Autodesk Inventor part; units mm, degrees
ref_plane "YZ Plane" through (0, 0, 0) normal (1, 0, 0) x (0, 1, 0)
ref_plane "XZ Plane" through (0, 0, 0) normal (0, 1, 0) x (-1, 0, 0)
ref_plane "XY Plane" through (0, 0, 0) normal (0, 0, 1) x (1, 0, 0)
sketch "Sketch1" plane through (0, 0, 0) normal (0, 1, 0) x (-1, 0, 0)
  line L0 (0, 0) -> (-25.4, 0)
  line L1 (-25.4, 0) -> (-25.4, 25.4)
  line L2 (-25.4, 25.4) -> (0, 25.4)
  line L3 (0, 25.4) -> (0, 0)
  line L4 (-1.5875, 23.8125) -> (-23.8125, 23.8125)
  line L5 (-23.8125, 23.8125) -> (-23.8125, 1.5875)
  line L6 (-23.8125, 1.5875) -> (-1.5875, 1.5875)
  line L7 (-1.5875, 1.5875) -> (-1.5875, 23.8125)
  dimension "d0" = 25.4
  dimension "d2" = 25.4
  dimension "d3" = 1.5875
extrude "Extrusion1" add sketch "Sketch1" along normal blind 593.725
sketch "Sketch5" plane through (25.4, 0, 25.4) normal (1, 0, 0) x (0, 0, -1)
  circle A0 centre (12.7, 561.975) radius 3.3782
  circle A1 centre (12.7, 539.75) radius 3.3782
  circle A2 centre (12.7, 454.025) radius 3.3782
extrude "Cut3" cut sketch "Sketch5" against normal blind 2540
sketch "Sketch6" plane through (0, 0, 25.4) normal (0, 0, 1) x (1, 0, 0)
  circle A0 centre (12.7, 428.625) radius 3.3782
  circle A1 centre (12.7, 377.825) radius 3.3782
  circle A2 centre (12.7, 571.5) radius 3.3782
  circle A3 centre (12.7, 549.275) radius 3.3782
extrude "Cut4" cut sketch "Sketch6" against normal blind 2540
equation "\"BendRadius\" = Thickness"
equation "\"BendReliefWidth\" = Thickness"
equation "\"BendReliefDepth\" = 0.5 * Thickness"
equation "\"CornerReliefSize\" = 4 * Thickness"
equation "\"MinimumRemnant\" = 2 * Thickness"
equation "\"TransitionRadius\" = BendRadius"
equation "\"JacobiRadiusSize\" = Thickness"
equation "\"GapSize\" = Thickness"
properties part number "edge mount shortened" material "Aluminum 6061"
Verification items for the finished model (mm, model axes). A direction names the side the tool comes from. Round coordinates to 2 decimals unless told otherwise and drop trailing zeros. Write each loop counter-clockwise with the first axis right and the second up, starting at its lowest first coordinate (ties: lowest second). Pieces come first, ordered by that corner, then holes. Notation, with made-up numbers: (20, 39) -> (77, 39) arc R9 ccw to (77, 47) -> close; hole circle Ø2 at (-12, 42.25). An arc over 180 degrees is marked (long way). Write each question's results on one line, items separated by ' | '. Start each with the question number.
1. Depth check by flat-ended pin: P1, Ø5, axis at y = 372.5, z = 4.5, coming from the -X side. Enter the tip coordinate at first touch or a pass-through.
2. Set-up check for faces 4 (the flat face through (23.812, 293, 13)), 5 (the flat face through (13, 293, 0)): record each of +Z, -Z, +X, -X, +Y, -Y from which the full face is reachable in a straight line by a thin tool's end or side.
3. Cross-section at A-A (y = 189.5). Enter the section's corners in (x, z), then the cut area to 3 significant figures.
4. Draft check along X on faces 1 (the flat face through (0, 293, 13)), 2 (the flat face through (1.588, 293, 13)), 3 (the flat face through (24, 593.725, 13)). Enter one of: +X half, -X half, draft (parallel to the pull), parting line (faces both ways), or undercut.
5. Material ranges on probe 1 along Y at (x, z) = (24.75, 12.7) (3 decimals); probe 2 along Y at (x, z) = (12.7, 24.3) (3 decimals); probe 3 along X at (y, z) = (295, 20.5), recorded low to high. Write a range as from..to.
Solutions:
1) P1: stops at x = 0
2) face 4: +Y, -Y | face 5: -Z, +X, -X, +Y, -Y
3) outline: (0, 0) -> (25.4, 0) -> (25.4, 25.4) -> (0, 25.4) -> close; hole (1.59, 1.59) -> (23.81, 1.59) -> (23.81, 23.81) -> (1.59, 23.81) -> close | area: 151 mm2
4) face 1: -X half | face 2: undercut | face 3: draft
5) probe 1: y = 0..450.647, 457.403..536.372, 543.128..558.597, 565.353..593.725 | probe 2: y = 0..374.447, 381.203..425.247, 432.003..545.897, 552.653..568.122, 574.878..593.725 | probe 3: x = 0..1.59, 23.81..25.4
